from build123d import *

# Parameters (mm, degrees)
F0_W     = 106.8777292967
F0_H     = 43.1794375181
F1_DEPTH = 80.772
F2_T     = -2.54
F3_W     = 106.1705686152
F3_H     = 77.9809653759
F4_DEPTH = 33.782
F5_T     = -2.54


# Not quite as in the source:
# - a shell that OpenCascade refuses in one call is made with other operations: the cavity is built on its own and cut out


with BuildPart() as f1:
    # F0 (on Front) → F1 (new body)
    with BuildSketch(Plane.XZ):
        with Locations((-4.4315196574, 33.3908237517)):
            Rectangle(F0_W, F0_H)
    extrude(amount=F1_DEPTH)

    # F2
    f2_openings = [f1.faces().sort_by_distance(p)[0] for p in [
        (-4.43152, -40.386, 54.980543),
    ]]
    offset(amount=F2_T, openings=f2_openings)

    # F3 (on Top) → F4 (join)
    with BuildSketch(Plane.XY):
        with Locations((-15.3196584433, -118.8506782055)):
            Rectangle(F3_W, F3_H)
    extrude(amount=F4_DEPTH)

    # F5: a shell. OpenCascade refuses it in one call, so the cavity is built on its own and cut out:
    # the body offset inwards by the wall thickness, plus a prism from it out through each open face.
    f5_core = offset(f1.part, amount=F5_T, kind=Kind.INTERSECTION, mode=Mode.PRIVATE)
    f5_exits = [f5_core.faces().sort_by_distance(p)[0] for p in [
        (-15.216343, -118.119753, 31.242),
    ]]
    add(f5_core, mode=Mode.SUBTRACT)
    extrude(f5_exits, amount=-F5_T, mode=Mode.SUBTRACT)


solid = f1.part
Could you check a few things on this model? Use its own coordinates, in mm. A direction names the side the tool comes from. Give positions to 0.01 mm unless a question says otherwise; leave off trailing zeros. Order: outer loops, then holes, each group sorted by start corner. A loop starts at its lowest first (then second) coordinate and runs counter-clockwise, first axis right, second up.
Item 1: I'm going to push flat-ended pins straight in: pin 1 (3 mm diameter, centred on x = -8.5, y = -77, fed in from -Z); pin 2 (10 mm diameter, centred on x = -55.5, z = 29, fed in from +Y); pin 3 (22 mm diameter, centred on x = -9, y = -118, fed in from +Z); pin 4 (8 mm diameter, centred on y = -25.5, z = 23, fed in from -X). Where does each tip first touch, or does it pass through?
Item 2: I need wall thicknesses on line 1 (Y direction, x = -29, z = 18.5); line 2 (X direction, y = -31, z = 52.5); line 3 (X direction, y = -133.5, z = 10). Which ranges of each line are inside material? Lowest first, please.
Item 3: If we mould it in two halves opening along Y, with no side actions, what happens to faces 3 (the face through (46.467, -40, 34)), 4 (the face through (-16, -118, 0)), 5 (the face through (-5, 0, 34))? For each: pulls with the +Y half, pulls with the -Y half, needs draft (parallel to the pull), parting line crosses it, or undercut.
Item 4: If we section it at B-B, the plane y = -126.5: Write out the boundary of the cut face in (x, z), plus the area to 3 significant figures.
Item 5: For faces 1 (the face through (-5, -40, 14.341)), 2 (the face through (-16, -157.841, 17)), which set-ups out of +Z, -Z, +X, -X, +Y, -Y let a thin tool reach every point of the face, with its end or its side?
Item 6: If we section it at C-C, the plane x = 40: Write out the boundary of the cut face in (y, z), plus the area to 3 significant figures.
Item 7: If we section it at A-A, the plane z = 36: Write out the boundary of the cut face in (x, y), plus the area to 3 significant figures.
Item 8: If we section it at D-D, the plane z = 24: Write out the boundary of the cut face in (x, y).
Values:
1. pin 1: stops at z = 11.8
1. pin 2: stops at y = 0
1. pin 3: stops at z = 2.54
1. pin 4: stops at x = -57.87
2. line 1: y = -157.84 to -155.3, -80.77 to -78.23, -2.54 to 0
2. line 2: x = -57.87 to -55.33, 46.47 to 49.01
2. line 3: x = -68.4 to -65.86, 35.23 to 37.77
3. face 3: undercut
3. face 4: needs draft
3. face 5: pulls with the +Y half
4. outline: (-68.4, 0) - (37.77, 0) - (37.77, 33.78) - (35.23, 33.78) - (35.23, 2.54) - (-65.86, 2.54) - (-65.86, 33.78) - (-68.4, 33.78) - close
4. area: 428 mm2
5. face 1: +Z
5. face 2: +Z, -Z, +X, -X, -Y
6. outline: (-80.77, 11.8) - (0, 11.8) - (0, 54.98) - (-2.54, 54.98) - (-2.54, 14.34) - (-78.23, 14.34) - (-78.23, 54.98) - (-80.77, 54.98) - close
6. area: 412 mm2
7. outline: (-57.87, -80.77) - (49.01, -80.77) - (49.01, 0) - (-57.87, 0) - close; hole (-55.33, -78.23) - (46.47, -78.23) - (46.47, -2.54) - (-55.33, -2.54) - close
7. area: 927 mm2
8. outline: (-68.4, -157.84) - (37.77, -157.84) - (37.77, -80.77) - (49.01, -80.77) - (49.01, 0) - (-57.87, 0) - (-57.87, -79.86) - (-68.4, -79.86) - close; hole (-65.86, -155.3) - (35.23, -155.3) - (35.23, -80.77) - (-55.33, -80.77) - (-55.33, -82.4) - (-65.86, -82.4) - close; hole (-55.33, -78.23) - (46.47, -78.23) - (46.47, -2.54) - (-55.33, -2.54) - close
